Work out the finished part from the listing and answer in its coordinate system (mm). A direction names the side the tool comes from. Give positions to 0.01 mm unless a question says otherwise; leave off trailing zeros. Loops run counter-clockwise (first coordinate to the right, second up) from the corner with the lowest first, then second, coordinate; pieces in that order, holes last. Notation, with made-up numbers: M 45,34 L 98,34 A25 ccw 98,52 Z; hole C 60,14 d11. An arc over 180 degrees is marked long. Use a Markdown table: item, result.
```python
from build123d import *

# Parameters (mm, degrees)
F1_DEPTH = 730.25
F2_DEPTH = 6.35


with BuildPart() as f1:
    # F0 (on Top) → F1 (new body)
    with BuildSketch(Plane.XY):
        Polygon((-290.32869, 56.021555), (-290.32869, 30.621555), (-264.92869, 30.621555), (-264.92869, 33.796555), (-287.15369, 33.796555), (-287.15369, 56.021555), align=None)
    extrude(amount=-F1_DEPTH)

    # F1_face (on face) → F2 (join)
    with BuildSketch(Plane(origin=(-282.814523, 38.135722, 0), x_dir=(1, 0, 0), z_dir=(0, 0, 1))):
        Polygon((-7.514167, 17.885833), (-7.514167, -7.514167), (17.885833, -7.514167), (17.885833, -4.339167), (-4.339167, -4.339167), (-4.339167, 17.885833), align=None)
    extrude(amount=F2_DEPTH)


solid = f1.part
```
(1) A cutting plane is placed at A-A (z = -598). Write down the section's boundary in (x, y), and give its area (3 significant figures).
Entries:
| item | result |
|---|---|
| outline | M -290.33,30.62 L -264.93,30.62 L -264.93,33.8 L -287.15,33.8 L -287.15,56.02 L -290.33,56.02 Z |
| area | 151 mm² |
(2) A cutting plane is placed at B-B (x = -271.25). Write down the section's boundary in (y, z), and give its area (3 significant figures).
Entries:
| item | result |
|---|---|
| outline | M 30.62,-730.25 L 33.8,-730.25 L 33.8,6.35 L 30.62,6.35 Z |
| area | 2,340 mm² |
(3) Given P1, Ø5, axis at x = -284, y = 48.5, coming from the +Z side; P2, Ø12, axis at x = -285.5, z = -449.5, coming from the +Y side; P3, Ø3, axis at y = 44.5, z = -487.5, coming from the +X side; P4, Ø11, axis at x = -281.5, z = -463, coming from the +Y side, each flat-ended and moving along its own axis, determine where each tip first touches the part or whether it passes through.
Entries:
| item | result |
|---|---|
| P1 | passes through |
| P2 | stops at y = 56.02 |
| P3 | stops at x = -287.15 |
| P4 | stops at y = 33.8 |
(4) Consider probe 1 along Y at (x, z) = (-281.5, -472); probe 2 along X at (y, z) = (40, -421). Determine where each line is inside the solid, lowest interval first. Write a range as [from, to].
Entries:
| item | result |
|---|---|
| probe 1 | y = [30.62, 33.8] |
| probe 2 | x = [-290.33, -287.15] |
(5) A cutting plane is placed at C-C (y = 41). Write down the section's boundary in (x, z).
Entries:
| item | result |
|---|---|
| outline | M -290.33,-730.25 L -287.15,-730.25 L -287.15,6.35 L -290.33,6.35 Z |
(6) Which of the six approach directions +Z, -Z, +X, -X, +Y, -Y give full straight-line access (tool end or side, diameter ignored) to faces 1 (the flat face through (-276, 33.797, -367)), 2 (the flat face through (-283, 33, -730.25))?
Entries:
| item | result |
|---|---|
| face 1 | +Z, -Z, +X, +Y |
| face 2 | -Z, +X, -X, +Y, -Y |
